```python
from build123d import *

# Parameters (mm, degrees)
ESBO_O1_R                = 21
RESSALTO_EXTRUS_O1_DEPTH = 3
CORTE_EXTRUS_O1_DEPTH    = 30.849623113
PADR_OCIRCULAR1_COUNT    = 20
ESBO_O7_R                = 6
RESSALTO_EXTRUS_O2_DEPTH = 10
CHANFRO1_SIZE            = 3
ESBO_O8_R                = 1.3
CORTE_EXTRUS_O3_DEPTH    = 12


with BuildPart() as part:
    # Esboço1 → Ressalto-extrusão1 (new body)
    with BuildSketch(Plane.XY):
        Circle(ESBO_O1_R)
    extrude(amount=RESSALTO_EXTRUS_O1_DEPTH)

    # Esboço5 → Corte-extrusão1 (cut, through all)
    with BuildSketch(Plane.XY.offset(3)):
        with BuildLine():
            Line((-0.501622955, 11.489054548), (-0.850578054, 19.481440321))
            ThreePointArc((-0.850578054, 19.481440321), (0, 19.5), (0.850578054, 19.481440321))
            Line((0.850578054, 19.481440321), (0.501622955, 11.489054548))
            ThreePointArc((0.501622955, 11.489054548), (0, 11.5), (-0.501622955, 11.489054548))
        make_face()
    corte_extrus_o1 = extrude(amount=-CORTE_EXTRUS_O1_DEPTH, mode=Mode.SUBTRACT)

    # PadrãoCircular1: Corte-extrusão1 ×20 about axis
    padr_ocircular1_axis = Axis((0, 0, 0), (0, 0, 1))
    for i in range(1, PADR_OCIRCULAR1_COUNT):
        add(corte_extrus_o1.rotate(padr_ocircular1_axis, i * 360 / PADR_OCIRCULAR1_COUNT), mode=Mode.SUBTRACT)

    # Esboço7 → Ressalto-extrusão2 (add)
    with BuildSketch(Plane(origin=(0, 0, 0), x_dir=(-1, 0, 0), z_dir=(0, 0, -1))):
        with Locations(Location((0, 0, 0), (0, 0, 180))):
            Circle(ESBO_O7_R)
    extrude(amount=RESSALTO_EXTRUS_O2_DEPTH)

    # Chanfro1
    chanfro1_edges = [part.edges().sort_by_distance(p)[0] for p in [
        (-6, 0, -10),
    ]]
    chamfer(chanfro1_edges, length=CHANFRO1_SIZE)

    # Esboço8 → Corte-extrusão3 (cut)
    with BuildSketch(Plane(origin=(0, 0, -10), x_dir=(-1, 0, 0), z_dir=(0, 0, -1))):
        Circle(ESBO_O8_R)
    extrude(amount=-CORTE_EXTRUS_O3_DEPTH, mode=Mode.SUBTRACT)


solid = part.part
```
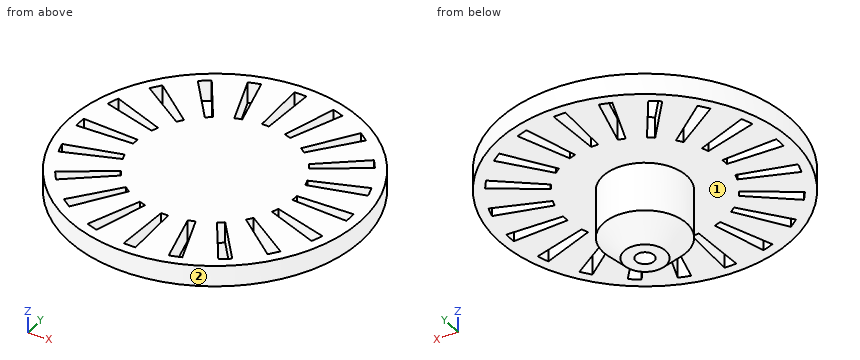
Design review of the part built by this model. Coordinates are the model's own, in mm. Face numbers are marked on the shaded views. A direction names the side the tool comes from. Coordinates: 2 decimals unless noted, no trailing zeros. Loops run counter-clockwise (first coordinate to the right, second up) from the corner with the lowest first, then second, coordinate; pieces in that order, holes last.
Q1. For pin 1 (1.5 mm diameter, centred on x = 12.5, y = 0, fed in from -Z); pin 2 (1.5 mm diameter, centred on y = -2, z = 0.5, fed in from +X); pin 3 (4 mm diameter, centred on y = 12, z = -1.5, fed in from +X), all flat-tipped, find the tip position at first contact; note any pin that passes through.
Reported:
pin 1: stops at z = 0
pin 2: stops at x = 20.96
pin 3: stops at x = 18.08
Q2. We need section A-A on y = 0. State the section outline as (x, z) points.
Reported:
outline: (-21, 0) - (-19.5, 0) - (-19.5, 3) - (-21, 3) - close; (-11.5, 0) - (-6, 0) - (-6, -7) - (-3, -10) - (-1.3, -10) - (-1.3, 2) - (1.3, 2) - (1.3, -10) - (3, -10) - (6, -7) - (6, 0) - (11.5, 0) - (11.5, 3) - (-11.5, 3) - close; (19.5, 0) - (21, 0) - (21, 3) - (19.5, 3) - close
Q3. Tool access review of the marked faces 1 and 2: name each direction out of +Z, -Z, +X, -X, +Y, -Y from which nothing blocks a thin tool from reaching the whole face with its end or side.
Reported:
face 1: -Z
face 2: +Z, -Z
Q4. We need section B-B on x = -17. State the section outline as (y, z) points, and give its area (3 significant figures).
Reported:
outline: (-12.33, 0) - (-6.36, 0) - (-6.36, 3) - (-12.33, 3) - close; (-4.71, 0) - (-0.74, 0) - (-0.74, 3) - (-4.71, 3) - close; (0.74, 0) - (4.71, 0) - (4.71, 3) - (0.74, 3) - close; (6.36, 0) - (12.33, 0) - (12.33, 3) - (6.36, 3) - close
area: 59.7 mm2
Q5. We need section D-D on z = -1. State the section outline as (x, y) points.
Reported:
outline: circle Ø12 at (0, 0); hole circle Ø2.6 at (0, 0)
Q6. To check wall thickness, follow line 1 (Y direction, x = 0, z = -1.75); line 2 (Y direction, x = 18, z = 2); line 3 (Z direction, x = 9.5, y = 18.5). State the ranges of each line that lie inside material, in increasing order.
Reported:
line 1: y = -6 to -1.3, 1.3 to 6
line 2: y = -10.82 to -6.73, -4.99 to -0.79, 0.79 to 4.99, 6.73 to 10.82
line 3: z = 0 to 3
